```python
from build123d import *

# Parameters (mm, degrees)
BOSS_EXTRUDE1_DEPTH = 100
CUT_EXTRUDE1_DEPTH  = 30
CUT_EXTRUDE2_DEPTH  = 40
SKETCH5_W           = 30
SKETCH5_H           = 40
CUT_EXTRUDE3_DEPTH  = 188.082869339


with BuildPart() as part:
    # Sketch1 → Boss-Extrude1 (new body)
    with BuildSketch(Plane.XY):
        Polygon((1.371761587, 0), (150, 0), (150, 40), (80, 80), (0, 80), align=None)
    extrude(amount=-BOSS_EXTRUDE1_DEPTH)

    # Sketch2 → Cut-Extrude1 (cut)
    with BuildSketch(Plane.XY):
        Polygon((0, 80), (0.514410595, 50), (50.514410595, 50), (50.514410595, 80), align=None)
    extrude(amount=-CUT_EXTRUDE1_DEPTH, mode=Mode.SUBTRACT)

    # Sketch3 → Cut-Extrude2 (cut)
    with BuildSketch(Plane(origin=(0, 0, -100), x_dir=(-1, 0, 0), z_dir=(0, 0, -1))):
        Polygon((0, 80), (-30.514410595, 80), (-30.514410595, 50), (-0.514410595, 50), align=None)
    extrude(amount=-CUT_EXTRUDE2_DEPTH, mode=Mode.SUBTRACT)

    # Sketch5 → Cut-Extrude3 (cut, through all)
    with BuildSketch(Plane(origin=(0, 50, 0), x_dir=(1, 0, 0), z_dir=(0, 1, 0))):
        with Locations((15.514410595, 80)):
            Rectangle(SKETCH5_W, SKETCH5_H)
    extrude(amount=-CUT_EXTRUDE3_DEPTH, mode=Mode.SUBTRACT)


solid = part.part
```
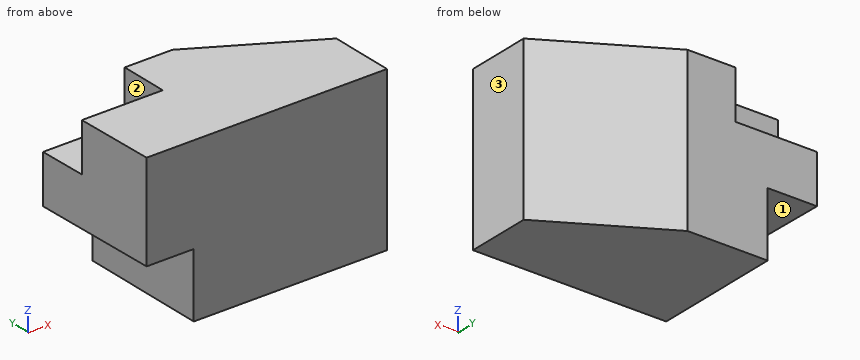
The model under review builds one solid part; all positions refer to its coordinate system, in mm. Face numbers are marked on the shaded views. A direction names the side the tool comes from. Round coordinates to 2 decimals unless told otherwise and drop trailing zeros. Loops run counter-clockwise (first coordinate to the right, second up) from the corner with the lowest first, then second, coordinate; pieces in that order, holes last. Notation, with made-up numbers: (17, -40) - (33, -40) arc R17 cw to (33, -9) - close; hole circle Ø3 at (48, 56). An arc over 180 degrees is marked (long way). Use a Markdown table: item, result. Add a question column.
Q1. Add section D-D (z = -56). State the section outline as (x, y) points.
Q2. For probe 1 along X at (y, z) = (18.5, -72); probe 2 along Z at (x, y) = (43, 67); probe 3 along X at (y, z) = (63, -63), list the stretches that pass through material, from the lowest coordinate up.
Q3. Add section C-C (x = 104.5). State the section outline as (y, z) points.
Q4. Insertion check: pin 1 Ø6 at (y, z) = (64, -41.5) entering from +X; pin 2 Ø8 at (x, z) = (133, -73) entering from +Y; pin 3 Ø24 at (x, y) = (33.5, 65) entering from +Z. Each pin has a flat end and moves straight along its axis. Give the tip position at first contact, or say it passes through.
Q5. Add section A-A (z = -12). State the section outline as (x, y) points.
Q6. Machinability: for the marked faces 1, 2 and 3, which of the approach directions +Z, -Z, +X, -X, +Y, -Y give a long, thin tool a straight path to every point of the face, cutting with its end or side? Answer none if there is none.
Q7. Add section B-B (y = 60.5). State the section outline as (x, z) points (3 decimals), plus the area to 3 significant figures.
Worked answers:
| question | item | result |
|---|---|---|
| 1 | outline | (0, 80) - (1.37, 0) - (150, 0) - (150, 40) - (80, 80) - close |
| 2 | probe 1 | 30.51 to 150 |
| 2 | probe 2 | -100 to -30 |
| 2 | probe 3 | 30.51 to 109.75 |
| 3 | outline | (0, -100) - (66, -100) - (66, 0) - (0, 0) - close |
| 4 | pin 1 | x = 113.25 |
| 4 | pin 2 | y = 52 |
| 4 | pin 3 | z = -30 |
| 5 | outline | (0.51, 50) - (1.37, 0) - (150, 0) - (150, 40) - (80, 80) - (50.51, 80) - (50.51, 50) - close |
| 6 | face 1 | -Z, -X, +Y, -Y |
| 6 | face 2 | +Z, -X, +Y |
| 6 | face 3 | +Z, -Z, +X, +Y, -Y |
| 7 | outline | (0.334, -60) - (30.514, -60) - (30.514, -100) - (114.125, -100) - (114.125, 0) - (50.514, 0) - (50.514, -30) - (0.334, -30) - close |
| 7 | area | 8,670 mm² |
